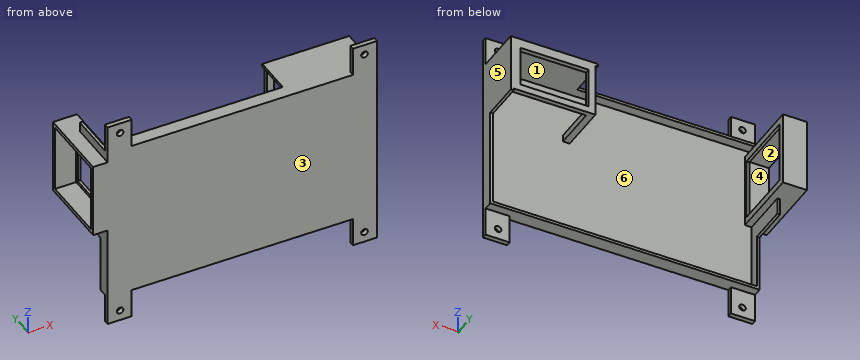
```python
from build123d import *

# Parameters (mm, degrees)
SKETCH1_W             = 280
SKETCH1_H             = 165.1
FLOOR_2_DEPTH         = 4
SKETCH2_W             = 280
SKETCH2_H             = 165.1
SKETCH2_W_2           = 274
SKETCH2_H_2           = 159.1
WALL_DEPTH            = 10
RPI_START             = 45
SKETCH4_W             = 85
SKETCH4_H             = 56
SKETCH4_W_2           = 71
SKETCH4_H_2           = 42
RPI_STAND_DEPTH       = 5
SKETCH7_W             = 3
SKETCH7_H             = 105.333904831
TEMP_SUPPORT_DEPTH    = 40
SKETCH3_W             = 25
SKETCH3_H             = 30
SKETCH3_R             = 3.429
BRACKETS_DEPTH        = 5
FAN_HOLDER_DEPTH      = 15
FAN_HOLDER_DEPTH_BACK = 10
SKETCH5_W             = 78
SKETCH5_H             = 78
SKETCH5_W_2           = 70
SKETCH5_H_2           = 70
SKETCH8_W             = 70
SKETCH8_H             = 50
FAN_HOLE_DEPTH        = 3
SKETCH11_W            = 78
SKETCH11_H            = 78
SKETCH11_W_2          = 64
SKETCH11_H_2          = 64
BOSS_EXTRUDE9_DEPTH   = 3
BOSS_EXTRUDE10_REACH  = 199.721
SKETCH12_W            = 7
SKETCH12_H            = 7


with BuildPart() as part:
    # Sketch1 → Floor 2 (new body)
    with BuildSketch(Plane(origin=(0, 0, 0), x_dir=(1, 0, 0), z_dir=(0, 1, 0))):
        Rectangle(SKETCH1_W, SKETCH1_H)
    extrude(amount=FLOOR_2_DEPTH)

    # Sketch2 → Wall (add)
    with BuildSketch(Plane(origin=(0, 4, 0), x_dir=(1, 0, 0), z_dir=(0, 1, 0))):
        Rectangle(SKETCH2_W, SKETCH2_H)
        Rectangle(SKETCH2_W_2, SKETCH2_H_2, mode=Mode.SUBTRACT)
    extrude(amount=WALL_DEPTH)

    # Sketch7 → Temp support (add)
    with BuildSketch(Plane(origin=(0, 14, 0), x_dir=(1, 0, 0), z_dir=(0, 1, 0))):
        with Locations((-138.5, -29.883047585)):
            Rectangle(SKETCH7_W, SKETCH7_H)
        Polygon((140, -82.55), (49.61228981, -82.55), (49.61228981, -79.55), (137, -79.55), (137, -21.306937857), (140, -21.306937857), (140, -79.55), align=None)
    extrude(amount=TEMP_SUPPORT_DEPTH)

    # Sketch3 → Brackets (add)
    # profile 1 of 4: a face of its own
    with BuildSketch(Plane(origin=(0, 0, 0), x_dir=(1, 0, 0), z_dir=(0, 1, 0))):
        with Locations((-127.5, 97.55)):
            Rectangle(SKETCH3_W, SKETCH3_H)
        with Locations(Location((-127, 101.6, 0), (0, 0, 270))):
            Circle(SKETCH3_R, mode=Mode.SUBTRACT)
    # profile 2 of 4: a face of its own
    with BuildSketch(Plane(origin=(0, 0, 0), x_dir=(1, 0, 0), z_dir=(0, 1, 0))):
        with Locations((127.5, 97.55)):
            Rectangle(SKETCH3_W, SKETCH3_H)
        with Locations(Location((127, 101.6, 0), (0, 0, 270))):
            Circle(SKETCH3_R, mode=Mode.SUBTRACT)
    # profile 3 of 4: a face of its own
    with BuildSketch(Plane(origin=(0, 0, 0), x_dir=(1, 0, 0), z_dir=(0, 1, 0))):
        with Locations((-127.5, -97.55)):
            Rectangle(SKETCH3_W, SKETCH3_H)
        with Locations(Location((-127, -101.6, 0), (0, 0, 270))):
            Circle(SKETCH3_R, mode=Mode.SUBTRACT)
    # profile 4 of 4: a face of its own
    with BuildSketch(Plane(origin=(0, 0, 0), x_dir=(1, 0, 0), z_dir=(0, 1, 0))):
        with Locations((127.5, -97.55)):
            Rectangle(SKETCH3_W, SKETCH3_H)
        with Locations(Location((127, -101.6, 0), (0, 0, 270))):
            Circle(SKETCH3_R, mode=Mode.SUBTRACT)
    extrude(amount=BRACKETS_DEPTH)

    # Sketch5 → Fan Holder (add, two sides: drawn at the far end of the back side and taken through both)
    with BuildSketch(Plane.ZY.offset(140).offset(-FAN_HOLDER_DEPTH_BACK)):
        with Locations((33.55, 39)):
            Rectangle(SKETCH5_W, SKETCH5_H)
        with Locations((33.55, 39)):
            Rectangle(SKETCH5_W_2, SKETCH5_H_2, mode=Mode.SUBTRACT)
    extrude(amount=FAN_HOLDER_DEPTH + FAN_HOLDER_DEPTH_BACK)

    # Sketch8 → Fan hole (cut)
    with BuildSketch(Plane.ZY.offset(140)):
        with Locations((33.55, 29)):
            Rectangle(SKETCH8_W, SKETCH8_H)
    extrude(amount=-FAN_HOLE_DEPTH, mode=Mode.SUBTRACT)

    # Sketch11 → Boss-Extrude9 (add)
    with BuildSketch(Plane.ZY.offset(130)):
        with Locations((33.55, 39)):
            Rectangle(SKETCH11_W, SKETCH11_H)
        with Locations((33.55, 39)):
            Rectangle(SKETCH11_W_2, SKETCH11_H_2, mode=Mode.SUBTRACT)
    extrude(amount=BOSS_EXTRUDE9_DEPTH)

    # Sketch12 → Boss-Extrude10 (add, up to next)
    with BuildSketch(Plane.XZ.offset(-49), mode=Mode.PRIVATE) as boss_extrude10_sk1:
        with Locations((55.5, 27.05)):
            Rectangle(SKETCH12_W, SKETCH12_H)
    boss_extrude10_tool1 = extrude(boss_extrude10_sk1.sketch, amount=BOSS_EXTRUDE10_REACH, mode=Mode.PRIVATE) - part.part


with BuildPart() as body_2:
    # Sketch4 → Rpi stand (new body)
    with BuildSketch(Plane(origin=(0, 4, 0), x_dir=(1, 0, 0), z_dir=(0, 1, 0)).offset(RPI_START)):
        with Locations((94.5, -51.55)):
            Rectangle(SKETCH4_W, SKETCH4_H)
        with Locations((94.5, -51.55)):
            Rectangle(SKETCH4_W_2, SKETCH4_H_2, mode=Mode.SUBTRACT)
    extrude(amount=RPI_STAND_DEPTH)


with BuildPart() as part_1:
    add(part.part)

    add(body_2.part)  # Boss-Extrude10 merges body 2
    add(boss_extrude10_tool1.solids().sort_by_distance((55.5, 49, 27.05))[0])


solid = part_1.part
```
Design review of the part built by this model. Coordinates are the model's own, in mm. Face numbers are marked on the shaded views. A direction names the side the tool comes from. Give positions to 0.01 mm unless a question says otherwise; leave off trailing zeros. Write each loop counter-clockwise with the first axis right and the second up, starting at its lowest first coordinate (ties: lowest second). Pieces come first, ordered by that corner, then holes. Notation, with made-up numbers: (9.5, -30.5) - (43.5, -30.5) arc R25 cw to (43.5, 7.5) - close; hole circle Ø7 at (-4, 38). An arc over 180 degrees is marked (long way). Return JSON: item names as keys, results as strings. Group by question number.
(1) Insertion check: pin 1 (3 mm diameter, centred on x = 21.5, z = 84.5, fed in from +Y); pin 2 (3.5 mm diameter, centred on x = -138.5, z = -10, fed in from +Y); pin 3 (4 mm diameter, centred on x = -44, y = 8.5, fed in from -Z); pin 4 (11 mm diameter, centred on x = -145, z = 26.5, fed in from -Y). Each pin has a flat end and moves straight along its axis. Give the tip position at first contact, or say it passes through.
(2) We need section C-C, the plane x = 14. Give the boundary of the cut face in (y, z).
(3) Mouldability with a two-part tool opening along X and no side actions: class the marked faces 4, 5 and 6 as +X half, -X half, draft (parallel to the pull), parting line (faces both ways), or undercut.
(4) We need section A-A, the plane z = 15. Give the boundary of the cut face in (x, y), then the cut area to 3 significant figures.
(5) We need section D-D, the plane y = 35.5. Give the number of separate pieces and of enclosed holes in the cut face, then the cut area to 3 significant figures.
(6) We need section B-B, the plane z = 101.6. Give the boundary of the cut face in (x, y), then the cut area to 3 significant figures.
(7) To check wall thickness, follow probe 1 along X at (y, z) = (1, 101); probe 2 along X at (y, z) = (12.5, 29.5); probe 3 along Z at (x, y) = (-38.5, 6). State the ranges of each line that lie inside material, in increasing order.
(8) Machinability: for the marked faces 1, 2 and 3, which of the approach directions +Z, -Z, +X, -X, +Y, -Y give a long, thin tool a straight path to every point of the face, cutting with its end or side? Answer none if there is none.
Reported:
{
 "1": {"pin 1": "passes through", "pin 2": "stops at y = 54", "pin 3": "stops at z = -82.55", "pin 4": "stops at y = 0"},
 "2": {"outline": "(0, -82.55) - (14, -82.55) - (14, -79.55) - (4, -79.55) - (4, 79.55) - (14, 79.55) - (14, 82.55) - (0, 82.55) - close"},
 "3": {"face 4": "draft", "face 5": "+X half", "face 6": "undercut"},
 "4": {"outline": "(-155, 0) - (140, 0) - (140, 14) - (137, 14) - (137, 4) - (-130, 4) - (-130, 7) - (-133, 7) - (-133, 4) - (-155, 4) - close; (-155, 74) - (-133, 74) - (-133, 71) - (-130, 71) - (-130, 78) - (-155, 78) - close", "area": "1,330 mm2"},
 "5": {"separate pieces": "4", "enclosed holes": "0", "area": "795 mm2"},
 "6": {"outline": "(-140, 0) - (-130.43, 0) - (-130.43, 5) - (-140, 5) - close; (-123.57, 0) - (-115, 0) - (-115, 5) - (-123.57, 5) - close; (115, 0) - (123.57, 0) - (123.57, 5) - (115, 5) - close; (130.43, 0) - (140, 0) - (140, 5) - (130.43, 5) - close", "area": "181 mm2"},
 "7": {"probe 1": "x = -140 to -130.38, -123.62 to -115, 115 to 123.62, 130.38 to 140", "probe 2": "x = 52 to 59, 137 to 140", "probe 3": "z = -82.55 to -79.55, 79.55 to 82.55"},
 "8": {"face 1": "none", "face 2": "-X", "face 3": "+Z, -Z, +X, -X, -Y"}
}
